from build123d import *

# Parameters (mm, degrees)
SKETCH1_R                  = 200.533
SKETCH1_R_2                = 104.775
BOSS_EXTRUDE1_DEPTH        = 6.35
F_9_0_196_DIAMETER_HOLE1_D = 4.9784
SKETCH4_W                  = 50.8
SKETCH4_H                  = 9.525
CUT_EXTRUDE1_DEPTH         = 284.66757072
F_9_0_196_DIAMETER_HOLE2_D = 4.9784
FILLET1_R                  = 6.35
FILLET2_R                  = 6.35


with BuildPart() as part:
    # Sketch1 → Boss-Extrude1 (new body)
    with BuildSketch(Plane(origin=(0, 0, 0), x_dir=(0, 1, 0), z_dir=(0, 0, 1))):
        with Locations(Location((0, 0, 0), (0, 0, 270))):
            Circle(SKETCH1_R)
        with Locations(Location((0, 0, 0), (0, 0, 270))):
            Circle(SKETCH1_R_2, mode=Mode.SUBTRACT)
    extrude(amount=BOSS_EXTRUDE1_DEPTH)

    # #9 (0.196) Diameter Hole1 (through all)
    with Locations(Plane.XY.offset(6.35)):
        with Locations((-96.774, 167.617484852), (-167.617484852, 96.774), (-193.548, 0), (-167.617484852, -96.774), (-96.774, -167.617484852), (0, -193.548), (96.774, -167.617484852), (167.617484852, -96.774), (193.548, 0), (167.617484852, 96.774), (96.774, 167.617484852), (0, 193.548)):
            Hole(F_9_0_196_DIAMETER_HOLE1_D / 2)

    # Sketch4 → Cut-Extrude1 (cut, through all)
    with BuildSketch(Plane.XY.offset(6.35)):
        with Locations((0, 106.3625)):
            Rectangle(SKETCH4_W, SKETCH4_H)
        with Locations((0, -106.3625)):
            Rectangle(SKETCH4_W, SKETCH4_H)
    extrude(amount=-CUT_EXTRUDE1_DEPTH, mode=Mode.SUBTRACT)

    # #9 (0.196) Diameter Hole2 (through all)
    with Locations(Plane.XY.offset(6.35)):
        with Locations((-114.3, 38.1), (-114.3, -38.1), (-38.1, -114.3), (38.1, -114.3), (114.3, -38.1), (114.3, 38.1), (38.1, 114.3), (-38.1, 114.3)):
            Hole(F_9_0_196_DIAMETER_HOLE2_D / 2)

    # Fillet1
    fillet1_edges = [part.edges().sort_by_distance(p)[0] for p in [
        (25.4, -101.649597269, 3.175),
        (-25.4, -101.649597269, 3.175),
        (-25.4, 101.649597269, 3.175),
        (25.4, 101.649597269, 3.175),
    ]]
    fillet(fillet1_edges, radius=FILLET1_R)

    # Fillet2
    fillet2_edges = [part.edges().sort_by_distance(p)[0] for p in [
        (25.4, -111.125, 3.175),
        (-25.4, -111.125, 3.175),
        (25.4, 111.125, 3.175),
        (-25.4, 111.125, 3.175),
    ]]
    fillet(fillet2_edges, radius=FILLET2_R)


solid = part.part
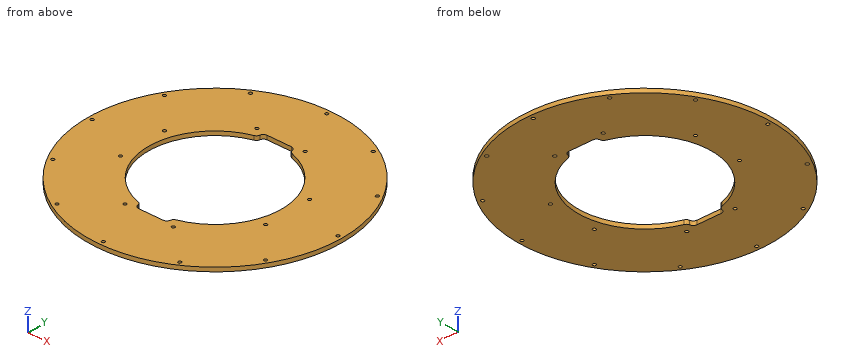
Verification items for the finished model (mm, model axes). Round coordinates to 2 decimals unless told otherwise and drop trailing zeros. Loops run counter-clockwise (first coordinate to the right, second up) from the corner with the lowest first, then second, coordinate; pieces in that order, holes last. Notation, with made-up numbers: (-15.75, 11.25) - (28.25, 11.25) arc R20 ccw to (28.25, 39.25) - close; hole circle Ø8 at (31, 70). An arc over 180 degrees is marked (long way). Use a Markdown table: item, result. Add a question column.
1. Gauge pin test, flat ends, axial feed: pin 1 (4.5 mm diameter, centred on x = 114.3, y = 38.1, fed in from -Z); pin 2 (2 mm diameter, centred on x = 98, z = 5.5, fed in from +Y); pin 3 (2 mm diameter, centred on x = -119.5, z = 4.5, fed in from -Y); pin 4 (1.9 mm diameter, centred on x = -4, z = 2.5, fed in from +Y). Record the tip position at first contact, or that the pin passes through.
2. Section check B-B, the plane y = 50.5. Record the boundary of the cut face in (x, z).
3. Thickness scan on probe 1 along Y at (x, z) = (0, 2) (3 decimals); probe 2 along X at (y, z) = (0.5, 4); probe 3 along Y at (x, z) = (38.1, 2). Record the ranges inside material, lowest first. Write a range as [from, to].
4. Section check A-A, the plane x = -61.5. Record the boundary of the cut face in (y, z), plus the area to 3 significant figures.
5. Section check C-C, the plane z = 3.5. Give the number of separate pieces and of enclosed holes in the cut face, plus the area to 3 significant figures.
Checks:
| question | item | result |
|---|---|---|
| 1 | pin 1 | passes through |
| 1 | pin 2 | stops at y = 175.51 |
| 1 | pin 3 | stops at y = -161.78 |
| 1 | pin 4 | stops at y = 200.51 |
| 2 | outline | (-194.07, 0) - (-91.8, 0) - (-91.8, 6.35) - (-194.07, 6.35) - close; (91.8, 0) - (194.07, 0) - (194.07, 6.35) - (91.8, 6.35) - close |
| 3 | probe 1 | y = [-200.533, -196.037], [-191.059, -111.125], [111.125, 191.059], [196.037, 200.533] |
| 3 | probe 2 | x = [-200.53, -195.99], [-191.11, -104.77], [104.77, 191.11], [195.99, 200.53] |
| 3 | probe 3 | y = [-196.88, -116.79], [-111.81, -97.6], [97.6, 111.81], [116.79, 196.88] |
| 4 | outline | (-190.87, 0) - (-84.83, 0) - (-84.83, 6.35) - (-190.87, 6.35) - close; (84.83, 0) - (190.87, 0) - (190.87, 6.35) - (84.83, 6.35) - close |
| 4 | area | 1,350 mm^2 |
| 5 | separate pieces | 1 |
| 5 | enclosed holes | 21 |
| 5 | area | 90,700 mm^2 |
